Could you check a few things on this drawing? It's one solid part, dimensions in mm from its lowest x, y, z. Give positions to 0.01 mm unless a question says otherwise; leave off trailing zeros. Loops run counter-clockwise (first coordinate to the right, second up) from the corner with the lowest first, then second, coordinate; pieces in that order, holes last. Notation, with made-up numbers: M 46,5.5 L 84,5.5 A18 cw 84,26.5 Z; hole C -8,-38.5 d1. An arc over 180 degrees is marked long. Answer as a JSON object with one key per item and string values.
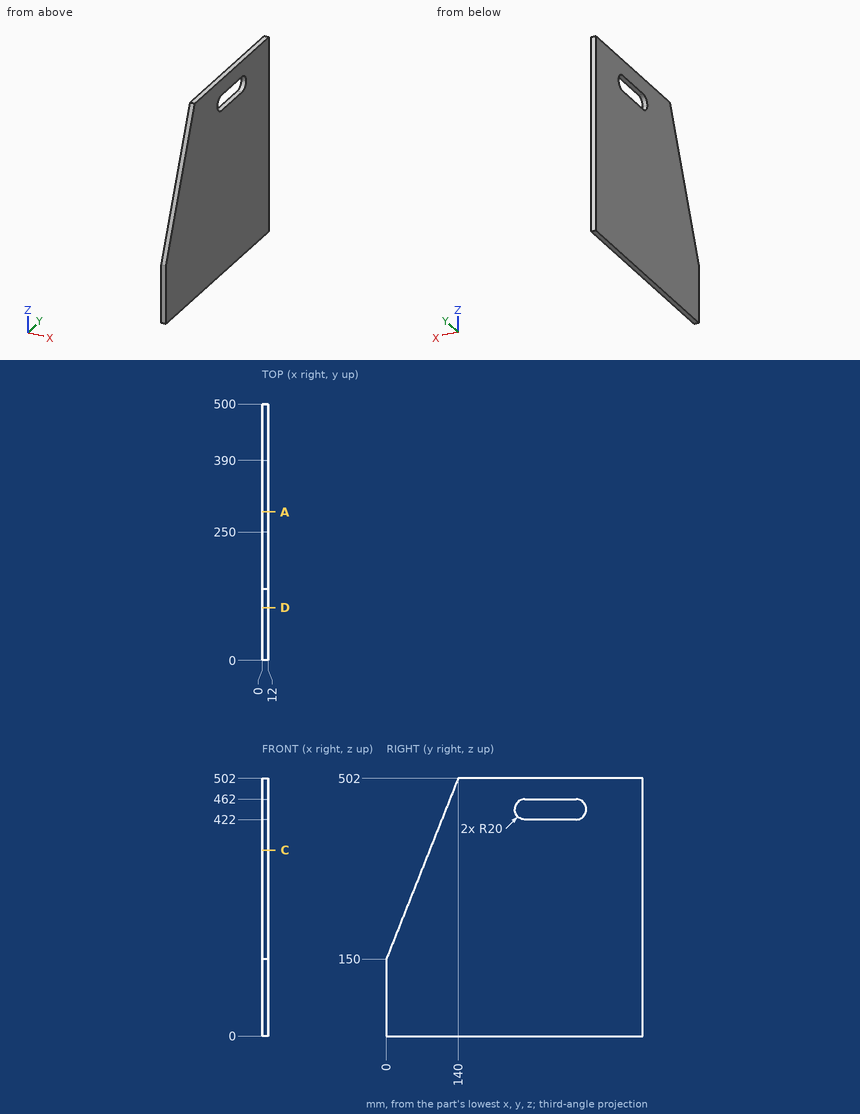
1) Will this pin go through, and if not, where does the flat tip stop? pin 1 Ø5 at (x, y) = (7.5, 66.5) entering from -Z.
Answer list:
{"pin 1": "z = 0"}
2) Please list where these lines run through material, in increasing order: line 1 along Z through (x, y) = (7.5, 331); line 2 along Z through (x, y) = (7, 381); line 3 along Y through (x, z) = (3.5, 341). Write a range as from..to.
Answer list:
{"line 1": "0..422, 462..502", "line 2": "0..425.3, 458.7..502", "line 3": "75.97..500"}
3) Suppose I cut it at D-D, the plane y = 103. Write out the boundary of the cut face in (x, z).
Answer list:
{"outline": "M 0,0 L 12,0 L 12,408.97 L 0,408.97 Z"}
4) Suppose I cut it at A-A, the plane y = 289.5. Write out the boundary of the cut face in (x, z), and give its area (3 significant figures).
Answer list:
{"outline": "M 0,0 L 12,0 L 12,422 L 0,422 Z; M 0,462 L 12,462 L 12,502 L 0,502 Z", "area": "5,540 mm^2"}
5) Suppose I cut it at C-C, the plane z = 362.5. Write out the boundary of the cut face in (x, y).
Answer list:
{"outline": "M 0,84.52 L 12,84.52 L 12,500 L 0,500 Z"}
